from build123d import *

# Parameters (mm, degrees)
F0_W          = 584.2
F0_H          = 584.2
F1_DEPTH      = 12.7
F2_W          = 584.2
F2_H          = 584.2
F2_W_2        = 558.8
F2_H_2        = 558.8
F3_DEPTH      = 152.4
F4_W          = 1017.536164
F4_H          = 883.057714
F4_W_2        = 558.8
F4_H_2        = 558.8
F5_DEPTH      = 508
F6_W          = 552.45
F6_H          = 552.45
F6_W_2        = 527.05
F6_H_2        = 527.05
F7_DEPTH      = 25.4
F8_W          = 584.2
F8_H          = 584.2
F8_W_2        = 552.45
F8_H_2        = 552.45
F9_DEPTH      = 12.7
F9_DEPTH_BACK = 25.4


with BuildPart() as f1:
    # F0 (on Top) → F1 (new body)
    with BuildSketch(Plane.XY):
        Rectangle(F0_W, F0_H)
    extrude(amount=F1_DEPTH)

    # F2 (on face) → F3 (join)
    with BuildSketch(Plane.XY.offset(12.7)):
        Rectangle(F2_W, F2_H)
        Rectangle(F2_W_2, F2_H_2, mode=Mode.SUBTRACT)
    extrude(amount=F3_DEPTH)

    # F4 (on face) → F5 (cut)
    with BuildSketch(Plane.XY.offset(12.7)):
        Rectangle(F4_W, F4_H)
        Rectangle(F4_W_2, F4_H_2, mode=Mode.SUBTRACT)
    extrude(amount=F5_DEPTH, mode=Mode.SUBTRACT)

    # F6 (on face) → F7 (join)
    with BuildSketch(Plane.XY.offset(12.7)):
        Rectangle(F6_W, F6_H)
        Rectangle(F6_W_2, F6_H_2, mode=Mode.SUBTRACT)
    extrude(amount=F7_DEPTH)

    # F8 (on face) → F9 (join, two sides)
    with BuildSketch(Plane.XY.offset(12.7)) as f9_sk:
        Rectangle(F8_W, F8_H)
        Rectangle(F8_W_2, F8_H_2, mode=Mode.SUBTRACT)
    extrude(amount=F9_DEPTH)
    extrude(f9_sk.sketch, amount=-F9_DEPTH_BACK)


solid = f1.part
For this review, take the finished solid that the model builds, in its own axes (mm). A direction names the side the tool comes from. Coordinates: 2 decimals unless noted, no trailing zeros. Write each loop counter-clockwise with the first axis right and the second up, starting at its lowest first coordinate (ties: lowest second). Pieces come first, ordered by that corner, then holes. Notation, with made-up numbers: (23, 23.25) -> (33, 23.25) arc R13 ccw to (33, 46.25) -> close; hole circle Ø9 at (-17.75, -22.75). An arc over 180 degrees is marked (long way). Write each question's results on one line, items separated by ' | '. Start each with the question number.
1) For faces 1 (the face through (-23, -280, -12.7)), 2 (the face through (-276.225, -4, 32)), 3 (the face through (276.225, -4, 32)), 4 (the face through (-4, 4, 12.7)), 5 (the face through (-4, -276.225, -6)), list the 3-axis set-ups (+Z, -Z, +X, -X, +Y, -Y) from which the entire face can be reached by the end or side of a thin tool; tool diameter is ignored.
2) Consider section A-A (x = -187). Write out the cut boundary in (y, z) (3 decimals), plus the area to 3 significant figures.
3) Insertion check: pin 1 (10 mm diameter, centred on x = -51.5, y = 10, fed in from +Z); pin 2 (3 mm diameter, centred on x = 228, y = 73.5, fed in from -Z); pin 3 (6.5 mm diameter, centred on y = 69, z = 34, fed in from +X) (3 decimals). Each pin has a flat end and moves straight along its axis. Give the tip position at first contact, or say it passes through.
4) Wall thickness on L1, parallel to X at y = 24, z = 24 (3 decimals); L2, parallel to Y at x = -134.5, z = -0.5 (3 decimals); L3, parallel to X at y = 189.5, z = 28.5 (3 decimals): over which ranges is each line inside the solid? List them lowest first. Write a range as [from, to].
5) The part is to be moulded in two halves that separate along Y. For faces 6 (the face through (-4, 4, 0)), 7 (the face through (-4, -292.1, 7)), 8 (the face through (-23, -280, 25.4)), 9 (the face through (-4, 263.525, 25)), say which applies: +Y half, -Y half, draft (parallel to the pull), parting line (faces both ways), or undercut.
Geometry says:
1) face 1: -Z, +X, -X, +Y, -Y | face 2: +Z, -X, +Y, -Y | face 3: +Z, +X, +Y, -Y | face 4: +Z | face 5: -Z
2) outline: (-292.1, -12.7) -> (-276.225, -12.7) -> (-276.225, 0) -> (276.225, 0) -> (276.225, -12.7) -> (292.1, -12.7) -> (292.1, 25.4) -> (276.225, 25.4) -> (276.225, 38.1) -> (263.525, 38.1) -> (263.525, 12.7) -> (-263.525, 12.7) -> (-263.525, 38.1) -> (-276.225, 38.1) -> (-276.225, 25.4) -> (-292.1, 25.4) -> close | area: 8,870 mm^2
3) pin 1: z = 12.7 | pin 2: z = 0 | pin 3: x = 276.225
4) L1: [-292.1, -263.525], [263.525, 292.1] | L2: [-292.1, -276.225], [276.225, 292.1] | L3: [-276.225, -263.525], [263.525, 276.225]
5) face 6: undercut | face 7: -Y half | face 8: draft | face 9: undercut
